from build123d import *

# Parameters (mm, degrees)
SKETCH_1_R          = 15
EXTRUDE_1_DEPTH     = 2.25
SKETCH_3_R          = 1
CUT_EXTRUDE_1_DEPTH = 5
SKETCH_4_R          = 3
CUT_EXTRUDE_2_DEPTH = 4.5


with BuildPart() as part:
    # ｽｹｯﾁ1 → ﾎﾞｽ - 押し出し1 (new, symmetric)
    with BuildSketch(Plane(origin=(0, 0, 0), x_dir=(1, 0, 0), z_dir=(0, 1, 0))):
        with Locations(Location((0, 0, 0), (0, 0, 270))):
            Circle(SKETCH_1_R)
    extrude(amount=EXTRUDE_1_DEPTH, both=True)

    # ｽｹｯﾁ3 → ｶｯﾄ - 押し出し1 (cut)
    with BuildSketch(Plane(origin=(0, 2.25, 0), x_dir=(1, 0, 0), z_dir=(0, 1, 0))):
        with Locations(Location((-11.382561056, -6.279912723, 0), (0, 0, 270))):
            Circle(SKETCH_3_R)
        with Locations(Location((-12.489254982, 3.608117238, 0), (0, 0, 270))):
            Circle(SKETCH_3_R)
        with Locations(Location((-6.279912723, 11.382561056, 0), (0, 0, 270))):
            Circle(SKETCH_3_R)
        with Locations(Location((3.608117238, 12.489254982, 0), (0, 0, 270))):
            Circle(SKETCH_3_R)
        with Locations(Location((11.382561056, 6.279912723, 0), (0, 0, 270))):
            Circle(SKETCH_3_R)
        with Locations(Location((12.489254982, -3.608117238, 0), (0, 0, 270))):
            Circle(SKETCH_3_R)
        with Locations(Location((6.279912723, -11.382561056, 0), (0, 0, 270))):
            Circle(SKETCH_3_R)
        with Locations(Location((-3.608117238, -12.489254982, 0), (0, 0, 270))):
            Circle(SKETCH_3_R)
    extrude(amount=-CUT_EXTRUDE_1_DEPTH, mode=Mode.SUBTRACT)

    # ｽｹｯﾁ4 → ｶｯﾄ - 押し出し2 (cut)
    with BuildSketch(Plane.XZ.offset(2.25)):
        with Locations(Location((0, 0, 0), (0, 0, 270))):
            Circle(SKETCH_4_R)
    extrude(amount=-CUT_EXTRUDE_2_DEPTH, mode=Mode.SUBTRACT)


solid = part.part
Here's how the part is built. I have some questions about the finished solid (model axes, mm). Round coordinates to 2 decimals unless told otherwise and drop trailing zeros. Order: outer loops, then holes, each group sorted by start corner. A loop starts at its lowest first (then second) coordinate and runs counter-clockwise, first axis right, second up. Notation, with made-up numbers: (-9, 74) -> (43, 74) arc R19 cw to (43, 97) -> close; hole circle Ø4 at (37.5, 85). An arc over 180 degrees is marked (long way). Return JSON: item names as keys, results as strings.
Q1. I need wall thicknesses on line 1 along X through (y, z) = (-0.15, -10.5); line 2 along Z through (x, y) = (2.5, 2.05); line 3 along Z through (x, y) = (6.75, 2). Which ranges of each line are inside material? Lowest first, please. Write a range as from..to.
Filled sheet:
{"line 1": "x = -10.71..-6.75, -5.81..10.71", "line 2": "z = -14.79..-1.66, 1.66..14.79", "line 3": "z = -13.4..10.5, 12.27..13.4"}
Q2. If we section it at C-C on y = -0.6: Give the number of separate pieces and of enclosed holes in the cut face, plus the area to 3 significant figures.
Filled sheet:
{"separate pieces": "1", "enclosed holes": "9", "area": "653 mm^2"}
Q3. If we mould it in two halves opening along X, with no side actions, what happens to faces 1 (the cylindrical face through (-13.465, 0.031, -3.825)), 2 (the cylindrical face through (0.66, 0.031, -14.985)), 3 (the flat face through (4, 2.25, 0))? For each: released by +X, released by -X, zero draft, split by the parting line, or undercut.
Filled sheet:
{"face 1": "undercut", "face 2": "split by the parting line", "face 3": "zero draft"}
Q4. If we section it at A-A on x = 0: List the corners of the cut face in (y, z) for me, plus the area to 3 significant figures.
Filled sheet:
{"outline": "(-2.25, -15) -> (2.25, -15) -> (2.25, -3) -> (-2.25, -3) -> close; (-2.25, 3) -> (2.25, 3) -> (2.25, 15) -> (-2.25, 15) -> close", "area": "108 mm^2"}
Q5. If we section it at B-B on z = 0: List the corners of the cut face in (x, y) for me, plus the area to 3 significant figures.
Filled sheet:
{"outline": "(-15, -2.25) -> (-3, -2.25) -> (-3, 2.25) -> (-15, 2.25) -> close; (3, -2.25) -> (15, -2.25) -> (15, 2.25) -> (3, 2.25) -> close", "area": "108 mm^2"}
Q6. For pin 1 Ø1 at (x, y) = (4, 0) entering from +Z, with a flat end and sliding along its axis, tell me the tip position at first contact or that it passes through.
Filled sheet:
{"pin 1": "stops at z = 14.59"}
Q7. If we section it at D-D on z = -9.5: List the corners of the cut face in (x, y) for me.
Filled sheet:
{"outline": "(-11.61, -2.25) -> (11.61, -2.25) -> (11.61, 2.25) -> (-11.61, 2.25) -> close"}
